The listing builds one solid part. Answer for the finished solid, in the listing's coordinates (mm). Face numbers are marked on the shaded views. A direction names the side the tool comes from. Give positions to 0.01 mm unless a question says otherwise; leave off trailing zeros. Write each loop counter-clockwise with the first axis right and the second up, starting at its lowest first coordinate (ties: lowest second). Pieces come first, ordered by that corner, then holes. Notation, with made-up numbers: (33.25, 16.5) -> (65.25, 16.5) arc R24 cw to (65.25, 44.5) -> close; hole circle Ø6 at (-20.75, 1.5). An arc over 180 degrees is marked (long way). Put each result on its own line as item: value. Start each with the question number.
1) Flat-ended cylindrical pins translate along their axes: pin 1 Ø1.2 at (x, z) = (0, 0) entering from +Y; pin 2 Ø2.5 at (x, z) = (-1, 0) entering from +Y; pin 3 Ø1 at (y, z) = (-0.5, -2) entering from -X; pin 4 Ø1.5 at (x, z) = (-16, -2) entering from +Y. Find the tip coordinate at first contact, or state that the pin passes through.
2) A cutting plane is placed at B-B (y = -1.35). Give the number of separate pieces and of enclosed holes in the cut face, then the cut area to 3 significant figures.
3) A cutting plane is placed at A-A (x = 0). Write down the section's boundary in (y, z) (3 decimals).
4) A cutting plane is placed at C-C (z = 3). Write down the section's boundary in (x, y), then the cut area to 3 significant figures.
5) Find the intervals of material crossed by line 1 along X through (y, z) = (-2, 0) (3 decimals); line 2 along Y through (x, z) = (-8, 1.5); line 3 along X through (y, z) = (2.05, -1.5), in increasing order. Write a range as from..to.
6) For the marked faces 1 and 2, determine the directions among +Z, -Z, +X, -X, +Y, -Y from which every point of the face is accessible in a straight line to the end or side of a thin tool.
7) For a pull along X with two mould halves and no side action, classify the marked faces 3, 4 and 5 as released by +X, released by -X, zero draft, split by the parting line, or undercut.
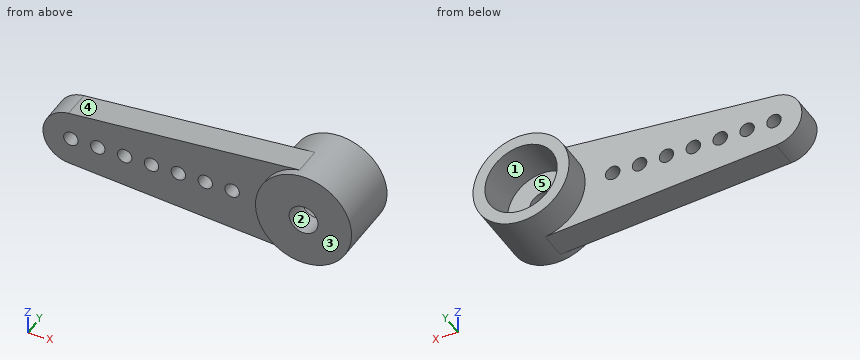
from build123d import *

# Parameters (mm, degrees)
SKETCH_1_R          = 3.325
EXTRUDE_1_DEPTH     = 2.34
SKETCH_2_R          = 2.5
CUT_EXTRUDE_1_DEPTH = 3
SKETCH_3_R          = 1
CUT_EXTRUDE_2_DEPTH = 6.577745961
EXTRUDE_2_DEPTH     = 2
SKETCH_5_R          = 0.5
CUT_EXTRUDE_3_DEPTH = 10


with BuildPart() as part:
    # 草图1 → 凸台-拉伸1 (new, symmetric)
    with BuildSketch(Plane(origin=(0, 0, 0), x_dir=(1, 0, 0), z_dir=(0, 1, 0))):
        with Locations(Location((0, 0, 0), (0, 0, 90))):
            Circle(SKETCH_1_R)
    extrude(amount=EXTRUDE_1_DEPTH, both=True)

    # 草图2 → 切除-拉伸1 (cut)
    with BuildSketch(Plane(origin=(0, 2.34, 0), x_dir=(1, 0, 0), z_dir=(0, 1, 0))):
        with Locations(Location((0, 0, 0), (0, 0, 270))):
            Circle(SKETCH_2_R)
    extrude(amount=-CUT_EXTRUDE_1_DEPTH, mode=Mode.SUBTRACT)

    # 草图3 → 切除-拉伸2 (cut, through all)
    with BuildSketch(Plane(origin=(0, -0.66, 0), x_dir=(1, 0, 0), z_dir=(0, 1, 0))):
        with Locations(Location((0, 0, 0), (0, 0, 270))):
            Circle(SKETCH_3_R)
    extrude(amount=-CUT_EXTRUDE_2_DEPTH, mode=Mode.SUBTRACT)

    # 草图4 → 凸台-拉伸2 (add)
    with BuildSketch(Plane(origin=(0, 0.22, 0), x_dir=(-1, 0, 0), z_dir=(0, -1, 0))):
        with BuildLine():
            Line((0, 3.325), (16.55, 1.92))
            ThreePointArc((16.55, 1.92), (18.325, 0), (16.55, -1.92))
            Line((16.55, -1.92), (0, -3.325))
            ThreePointArc((0, -3.325), (2.566190787, 0), (0, 3.325))
        make_face()
    extrude(amount=EXTRUDE_2_DEPTH)

    # 草图5 → 切除-拉伸3 (cut)
    with BuildSketch(Plane(origin=(0, -1.78, 0), x_dir=(-1, 0, 0), z_dir=(0, -1, 0))):
        with Locations(Location((14.535, 0, 0), (0, 0, 90))):
            Circle(SKETCH_5_R)
        with Locations(Location((16.395, 0, 0), (0, 0, 90))):
            Circle(SKETCH_5_R)
        with Locations(Location((12.675, 0, 0), (0, 0, 90))):
            Circle(SKETCH_5_R)
        with Locations(Location((10.815, 0, 0), (0, 0, 90))):
            Circle(SKETCH_5_R)
        with Locations(Location((8.955, 0, 0), (0, 0, 90))):
            Circle(SKETCH_5_R)
        with Locations(Location((7.095, 0, 0), (0, 0, 90))):
            Circle(SKETCH_5_R)
        with Locations(Location((5.235, 0, 0), (0, 0, 90))):
            Circle(SKETCH_5_R)
    extrude(amount=-CUT_EXTRUDE_3_DEPTH, mode=Mode.SUBTRACT)


solid = part.part
Reply:
1. pin 1: passes through
1. pin 2: stops at y = -0.66
1. pin 3: stops at x = -17.61
1. pin 4: stops at y = 0.22
2. separate pieces: 1
2. enclosed holes: 8
2. area: 101 mm2
3. outline: (-2.34, -3.325) -> (2.34, -3.325) -> (2.34, -2.5) -> (-0.66, -2.5) -> (-0.66, -1) -> (-2.34, -1) -> close; (-2.34, 1) -> (-0.66, 1) -> (-0.66, 2.5) -> (2.34, 2.5) -> (2.34, 3.325) -> (-2.34, 3.325) -> close
4. outline: (-3.83, -1.78) -> (-1.43, -1.78) -> (-1.43, -2.34) -> (1.43, -2.34) -> (1.43, 2.34) -> (-1.43, 2.34) -> (-1.43, 0.22) -> (-3.83, 0.22) -> close
4. area: 18.2 mm2
5. line 1: x = -3.325..-1, 1..3.325
5. line 2: y = -1.78..0.22
5. line 3: x = -2.97..-2, 2..2.97
6. face 1: +Y
6. face 2: +Y, -Y
7. face 3: zero draft
7. face 4: released by -X
7. face 5: undercut
